from build123d import *

# Parameters (mm, degrees)
SKETCH1_R           = 8.5
BOSS_EXTRUDE1_DEPTH = 6
FILLET2_R           = 1
SKETCH2_R           = 5
BOSS_EXTRUDE3_DEPTH = 6
BOSS_EXTRUDE3_TAPER = 2
FILLET4_R           = 1
BOSS_EXTRUDE4_START = 4
BOSS_EXTRUDE4_DEPTH = 4
CUT_EXTRUDE4_DEPTH  = 7


with BuildPart() as part:
    # Sketch1 → Boss-Extrude1 (new body)
    with BuildSketch(Plane(origin=(0, 0, 0), x_dir=(1, 0, 0), z_dir=(0, 1, 0))):
        with Locations(Location((-51.120170416, 0, 0), (0, 0, 270))):
            Circle(SKETCH1_R)
    extrude(amount=BOSS_EXTRUDE1_DEPTH)

    # Fillet2
    fillet2_edges = [part.edges().sort_by_distance(p)[0] for p in [
        (-51.120170416, 6, -8.5),
    ]]
    fillet(fillet2_edges, radius=FILLET2_R)

    # Sketch2 → Boss-Extrude3 (add)
    with BuildSketch(Plane(origin=(0, 6, 0), x_dir=(1, 0, 0), z_dir=(0, 1, 0))):
        with Locations((-51.120170416, 0)):
            Circle(SKETCH2_R)
    extrude(amount=BOSS_EXTRUDE3_DEPTH, taper=BOSS_EXTRUDE3_TAPER)

    # Fillet4
    fillet4_edges = [part.edges().sort_by_distance(p)[0] for p in [
        (-55.9106458, 12, 0),
    ]]
    fillet(fillet4_edges, radius=FILLET4_R)

    # Sketch3 → Boss-Extrude4 (add)
    with BuildSketch(Plane.XZ.offset(BOSS_EXTRUDE4_START)):
        with BuildLine():
            Line((-51.620170416, 0), (-59.620170416, 0))
            ThreePointArc((-59.620170416, 0), (-57.304828855, -5.830951895), (-51.620170416, -8.485281374))
            Line((-51.620170416, -8.485281374), (-51.620170416, 0))
        make_face()
        with BuildLine():
            ThreePointArc((-42.620170416, 0), (-51.120170416, 8.5), (-59.620170416, 0))
            Line((-59.620170416, 0), (-51.620170416, 0))
            Line((-51.620170416, 0), (-51.620170416, 1.514718626))
            Line((-51.620170416, 1.514718626), (-46.616547928, 1.514718626))
            Line((-46.616547928, 1.514718626), (-46.616547928, 0))
            Line((-46.616547928, 0), (-42.620170416, 0))
        make_face()
        with BuildLine():
            ThreePointArc((-46.616547928, -7.208840717), (-43.686100497, -4.121238215), (-42.620170416, 0))
            Line((-42.620170416, 0), (-46.616547928, 0))
            Line((-46.616547928, 0), (-46.616547928, -7.208840717))
        make_face()
    extrude(amount=-BOSS_EXTRUDE4_DEPTH)

    # Sketch6 → Cut-Extrude4 (cut)
    with BuildSketch(Plane.XZ.offset(4)):
        with BuildLine():
            ThreePointArc((-46.616547928, -7.208840717), (-49.019081783, -8.236226475), (-51.620170416, -8.485281374))
            Line((-51.620170416, -8.485281374), (-51.620170416, 1.514718626))
            Line((-51.620170416, 1.514718626), (-46.616547928, 1.514718626))
            Line((-46.616547928, 1.514718626), (-46.616547928, -7.208840717))
        make_face()
    extrude(amount=-CUT_EXTRUDE4_DEPTH, mode=Mode.SUBTRACT)


solid = part.part
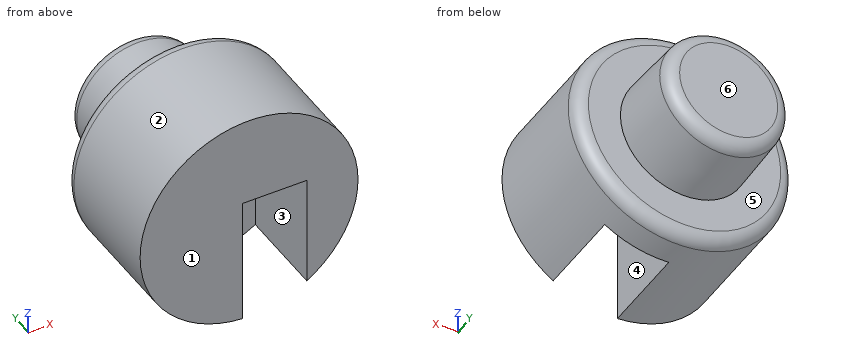
Work out the finished part from the listing and answer in its coordinate system (mm). Face numbers are marked on the shaded views. A direction names the side the tool comes from. Round coordinates to 2 decimals unless told otherwise and drop trailing zeros. Write each loop counter-clockwise with the first axis right and the second up, starting at its lowest first coordinate (ties: lowest second). Pieces come first, ordered by that corner, then holes.
1) Given pin 1 Ø2.5 at (x, y) = (-49.5, -1) entering from -Z; pin 2 Ø1 at (y, z) = (-0.5, 4) entering from -X; pin 3 Ø3 at (y, z) = (-2, -6.5) entering from -X; pin 4 Ø4 at (x, z) = (-48.5, -1.5) entering from -Y, each flat-ended and moving along its own axis, determine where each tip first touches the part or whether it passes through.
2) The mould has two halves that part along X. Classify the marked faces 1, 2 and 3: pulls with the +X half, pulls with the -X half, needs draft (parallel to the pull), parting line crosses it, or undercut.
3) A cutting plane is placed at A-A (y = 6.5). Give the vertices of the cut face in (x, z), plus the area to 3 significant figures.
4) A tool of negligible diameter and unlimited length cuts with its end or side. For the marked faces 4, 5 and 6, from which of +Z, -Z, +X, -X, +Y, -Y can it reach the whole face along a straight path? Write none if from no direction.
5) Straight lines are drawn through the part: line 1 (Z direction, x = -44.25, y = 1); line 2 (Z direction, x = -54, y = 11.25); line 3 (Y direction, x = -52, z = 7.5). For each, find the intervals that lie inside material, in ascending order.
Completed:
1. pin 1: stops at z = 1.51
1. pin 2: stops at x = -58.87
1. pin 3: stops at x = -57.99
1. pin 4: stops at y = -4
2. face 1: needs draft
2. face 2: parting line crosses it
2. face 3: undercut
3. outline: circle Ø9.97 at (-51.12, 0)
3. area: 78.0 mm2
4. face 4: -Z, -Y
4. face 5: +Y
4. face 6: +Z, -Z, +X, -X, +Y
5. line 1: z = -5.01 to 5.01
5. line 2: z = -3.83 to 3.83
5. line 3: y = -4 to 6
